Verification items for the finished model (mm, model axes). Round coordinates to 2 decimals unless told otherwise and drop trailing zeros. Order: outer loops, then holes, each group sorted by start corner. A loop starts at its lowest first (then second) coordinate and runs counter-clockwise, first axis right, second up. Notation, with made-up numbers: M 17,-12.75 L 74,-12.75 A18 ccw 74,20.25 Z; hole C 50.5,-8.75 d9. An arc over 180 degrees is marked long. One line per item, written item: value. Start each with the question number.
Autodesk Inventor part; units mm, degrees
ref_plane "YZ Plane" through (0, 0, 0) normal (1, 0, 0) x (0, 1, 0)
ref_plane "XZ Plane" through (0, 0, 0) normal (0, 1, 0) x (-1, 0, 0)
ref_plane "XY Plane" through (0, 0, 0) normal (0, 0, 1) x (1, 0, 0)
sketch "スケッチ1" plane through (0, 0, 0) normal (1, 0, 0) x (0, 1, 0)
  line L0 (0, 0) -> (-5, 0)
  line L1 (-5, 0) -> (-5, -30)
  line L2 (-5, -30) -> (0, -30)
  line L3 (0, -30) -> (0, 0)
  dimension "d0" = 30
  dimension "d1" = 5
extrude "押し出し1" add sketch "スケッチ1" along normal blind 280
sketch "スケッチ4" plane through (280, 0, -30) normal (0, 0, -1) x (-1, 0, 0)
  line L0 (280, 0) -> (0, 0)
  line L1 (280, -5) -> (280, 0)
  point P0 (260, -2.5)
  point P1 (40, -2.5)
  dimension "d27" = 2.5
  dimension "d28" = 20
  dimension "d36" = 220
hole "穴3" at (20, -2.5, -30) at (240, -2.5, -30) direction (0, 0, 1) diameter 2.459 end through all
sketch "スケッチ6" plane through (0, 0, 0) normal (0, 1, 0) x (1, 0, 0)
  line L0 (280, 30) -> (280, 0)
  line L1 (0, 0) -> (280, 0)
  point P0 (269, 13)
  dimension "d49" = 11
  dimension "d50" = 13
hole "穴5" at (269, 0, -13) direction (0, -1, 0) diameter 7 end through all
properties part number "横長2ndフラットバー" material "アルミニウム 6061"
1. Section check C-C (x = 269). Record the cut outline in (y, z), and give its area (3 significant figures).
2. Section check A-A (y = -2.5). Record the cut outline in (x, z).
3. Section check B-B (z = -13). Record the cut outline in (x, y), and give its area (3 significant figures).
4. Scan lines: line 1 along X through (y, z) = (-2.75, -13.25); line 2 along X through (y, z) = (-2.5, -7.5); line 3 along Y through (x, z) = (240, -21). Record each from-to range of solid material in increasing order.
5. Depth check by flat-ended pin: pin 1 (2 mm diameter, centred on x = 240, y = -2.5, fed in from +Z). Enter the tip coordinate at first touch or a pass-through.
Geometry check:
1. outline: M -5,-30 L 0,-30 L 0,-16.5 L -5,-16.5 Z; M -5,-9.5 L 0,-9.5 L 0,0 L -5,0 Z
1. area: 115 mm²
2. outline: M 0,-30 L 18.77,-30 L 18.77,0 L 0,0 Z; M 21.23,-30 L 238.77,-30 L 238.77,0 L 21.23,0 Z; M 241.23,-30 L 280,-30 L 280,0 L 241.23,0 Z; hole C 269,-13 d7
3. outline: M 0,-5 L 265.5,-5 L 265.5,0 L 0,0 Z; M 272.5,-5 L 280,-5 L 280,0 L 272.5,0 Z; hole C 20,-2.5 d2.46; hole C 240,-2.5 d2.46
3. area: 1,360 mm²
4. line 1: x = 0 to 18.8, 21.2 to 238.8, 241.2 to 265.51, 272.49 to 280
4. line 2: x = 0 to 18.77, 21.23 to 238.77, 241.23 to 280
4. line 3: y = -5 to -3.73, -1.27 to 0
5. pin 1: passes through
